```python
from build123d import *

# Parameters (mm, degrees)
SALIENTE_EXTRUIR1_START = 0.2
SALIENTE_EXTRUIR1_DEPTH = 21.6


with BuildPart() as part:
    # Croquis1 → Saliente-Extruir1 (new body)
    with BuildSketch(Plane(origin=(0, -0.153950711, 0), x_dir=(1, 0, 0), z_dir=(0, 1, 0)).offset(SALIENTE_EXTRUIR1_START)):
        with BuildLine():
            Line((-59.905314299, -154.5), (30.294685701, -154.5))
            Line((30.294685701, -154.5), (30.294685701, -153.55))
            Line((30.294685701, -153.55), (20.294685701, -153.55))
            Line((20.294685701, -153.55), (20.294685701, -152.75))
            Line((20.294685701, -152.75), (-60.155314299, -152.75))
            Line((-60.155314299, -152.75), (-60.155314299, -83.8))
            Line((-60.155314299, -83.8), (-60.905314299, -83.8))
            Line((-60.905314299, -83.8), (-60.905314299, -78.8))
            Line((-60.905314299, -78.8), (-61.905314299, -78.8))
            Line((-61.905314299, -78.8), (-61.905314299, -152.5))
            ThreePointArc((-61.905314299, -152.5), (-61.319527861, -153.914213562), (-59.905314299, -154.5))
        make_face()
    extrude(amount=SALIENTE_EXTRUIR1_DEPTH)


solid = part.part
```
Model file for the job. Use its own axes, mm. A direction names the side the tool comes from. Coordinates: 2 decimals unless noted, no trailing zeros. Write each loop counter-clockwise with the first axis right and the second up, starting at its lowest first coordinate (ties: lowest second). Pieces come first, ordered by that corner, then holes. Notation, with made-up numbers: (75.25, -37.75) - (90.25, -37.75) arc R25 ccw to (90.25, -3.75) - close; hole circle Ø7 at (-21, 55.25). An arc over 180 degrees is marked (long way). Use a Markdown table: item, result. Add a question column.
Item 1: Drill centre lines: line 1 along X through (y, z) = (11.5, 135); line 2 along Z through (x, y) = (-3, 13.5). Where is each one in solid material? Low to high.
Item 2: Band-saw the part on C-C, the plane z = 140. Write the cut outline in (x, y), and give its area (3 significant figures).
Item 3: Band-saw the part on A-A, the plane y = 13.25. Write the cut outline in (x, z), and give its area (3 significant figures).
Item 4: Band-saw the part on B-B, the plane x = -1. Write the cut outline in (y, z).
Item 5: 3-axis set-ups, long thin cutter, end or side, ignore diameter. For faces 1 (the face through (25, 11, 153.55)), 2 (the face through (-40, 21.646, 153)): which of +Z, -Z, +X, -X, +Y, -Y reach the whole face in a straight line?
Item 6: Drop flat-ended pins along their axis: pin 1 (10 mm diameter, centred on y = 18.5, z = 92, fed in from +X); pin 2 (3 mm diameter, centred on x = 25, y = 7.5, fed in from -Z); pin 3 (1.5 mm diameter, centred on x = -11.5, y = 10.5, fed in from -Z). Give the stop position or say it passes through.
A:
| question | item | result |
|---|---|---|
| 1 | line 1 | x = -61.91 to -60.16 |
| 1 | line 2 | z = 152.75 to 154.5 |
| 2 | outline | (-61.91, 0.05) - (-60.16, 0.05) - (-60.16, 21.65) - (-61.91, 21.65) - close |
| 2 | area | 37.8 mm² |
| 3 | outline | (-61.91, 78.8) - (-60.91, 78.8) - (-60.91, 83.8) - (-60.16, 83.8) - (-60.16, 152.75) - (20.29, 152.75) - (20.29, 153.55) - (30.29, 153.55) - (30.29, 154.5) - (-59.91, 154.5) arc R2 ccw to (-61.91, 152.5) - close |
| 3 | area | 278 mm² |
| 4 | outline | (0.05, 152.75) - (21.65, 152.75) - (21.65, 154.5) - (0.05, 154.5) - close |
| 5 | face 1 | -Z, +X, +Y, -Y |
| 5 | face 2 | +Z, -Z, +X, -X, +Y |
| 6 | pin 1 | stops at x = -60.16 |
| 6 | pin 2 | stops at z = 153.55 |
| 6 | pin 3 | stops at z = 152.75 |
